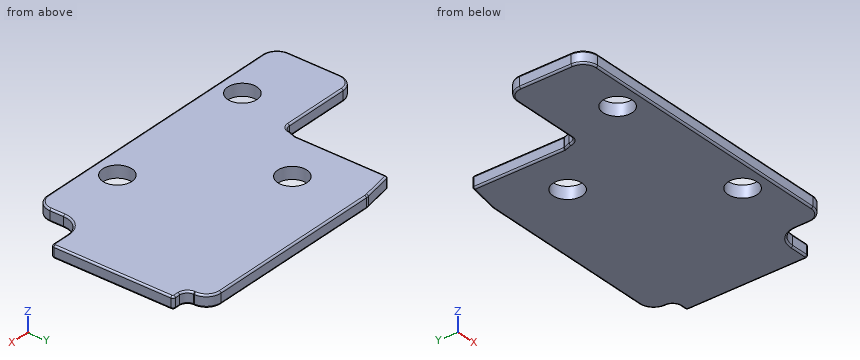
from build123d import *

# Parameters (mm, degrees)
SKETCH1_R           = 1.7
BOSS_EXTRUDE1_DEPTH = 1.4
FILLET1_R           = 0.2


with BuildPart() as part:
    # Sketch1 → Boss-Extrude1 (new body)
    with BuildSketch(Plane.XY):
        with BuildLine():
            Line((88.2, 306.15), (88.5, 306.997300304))
            Line((88.5, 306.997300304), (88.5, 317.666666667))
            Line((88.5, 317.666666667), (92.075260805, 318.322131148))
            ThreePointArc((92.075260805, 318.322131148), (92.227907414, 318.343018451), (92.381818182, 318.35))
            Line((92.381818182, 318.35), (113.2, 318.35))
            ThreePointArc((113.2, 318.35), (114.402081528, 317.852081528), (114.9, 316.65))
            Line((114.9, 316.65), (114.9, 316.55))
            ThreePointArc((114.9, 316.55), (115.163603897, 315.913603897), (115.8, 315.65))
            Line((115.8, 315.65), (116.4, 315.65))
            ThreePointArc((116.4, 315.65), (116.612132034, 315.562132034), (116.7, 315.35))
            Line((116.7, 315.35), (116.7, 301.75))
            ThreePointArc((116.7, 301.75), (116.612132034, 301.537867966), (116.4, 301.45))
            Line((116.4, 301.45), (114.4, 301.45))
            ThreePointArc((114.4, 301.45), (112.773654403, 300.776345597), (112.1, 299.15))
            Line((112.1, 299.15), (112.1, 297.55))
            ThreePointArc((112.1, 297.55), (111.602081528, 296.347918472), (110.4, 295.85))
            Line((110.4, 295.85), (79.6, 295.85))
            ThreePointArc((79.6, 295.85), (78.397918472, 296.347918472), (77.9, 297.55))
            Line((77.9, 297.55), (77.9, 303.55))
            ThreePointArc((77.9, 303.55), (78.397918472, 304.752081528), (79.6, 305.25))
            Line((79.6, 305.25), (87.3, 305.25))
            ThreePointArc((87.3, 305.25), (87.936396103, 305.513603897), (88.2, 306.15))
        make_face()
        with Locations((85.9, 298.65)):
            Circle(SKETCH1_R, mode=Mode.SUBTRACT)
        with Locations((103.8, 298.65)):
            Circle(SKETCH1_R, mode=Mode.SUBTRACT)
        with Locations((94, 311.05)):
            Circle(SKETCH1_R, mode=Mode.SUBTRACT)
    extrude(amount=BOSS_EXTRUDE1_DEPTH)

    # Fillet1
    fillet1_edges = [part.edges().sort_by_distance(p)[0] for p in [
        (88.35, 306.573650152, 1.4),
        (87.936396103, 305.513603897, 1.4),
        (83.45, 305.25, 1.4),
        (92.227907414, 318.343018451, 0),
        (102.790909091, 318.35, 0),
        (114.402081528, 317.852081528, 0),
        (114.9, 316.6, 0),
        (115.163603897, 315.913603897, 0),
        (116.1, 315.65, 0),
        (116.612132034, 315.562132034, 0),
        (116.7, 308.55, 0),
        (116.612132034, 301.537867966, 0),
        (115.4, 301.45, 0),
        (78.397918472, 304.752081528, 1.4),
        (112.773654403, 300.776345597, 0),
        (112.1, 298.35, 0),
        (111.602081528, 296.347918472, 0),
        (95, 295.85, 0),
        (78.397918472, 296.347918472, 0),
        (77.9, 300.55, 0),
        (78.397918472, 304.752081528, 0),
        (83.45, 305.25, 0),
        (87.936396103, 305.513603897, 0),
        (88.35, 306.573650152, 0),
        (77.9, 300.55, 1.4),
        (88.5, 312.331983485, 0),
        (90.287630402, 317.994398907, 0),
        (78.397918472, 296.347918472, 1.4),
        (95, 295.85, 1.4),
        (88.5, 306.997300304, 0.7),
        (88.5, 317.666666667, 0.7),
        (111.602081528, 296.347918472, 1.4),
        (112.1, 298.35, 1.4),
        (112.773654403, 300.776345597, 1.4),
        (90.287630402, 317.994398907, 1.4),
        (115.4, 301.45, 1.4),
        (116.612132034, 301.537867966, 1.4),
        (116.7, 308.55, 1.4),
        (116.612132034, 315.562132034, 1.4),
        (116.1, 315.65, 1.4),
        (115.163603897, 315.913603897, 1.4),
        (114.9, 316.6, 1.4),
        (114.402081528, 317.852081528, 1.4),
        (102.790909091, 318.35, 1.4),
        (92.227907414, 318.343018451, 1.4),
        (88.5, 312.331983485, 1.4),
    ]]
    fillet(fillet1_edges, radius=FILLET1_R)


solid = part.part
Could you check a few things on this model? Use its own coordinates, in mm. Give positions to 0.01 mm unless a question says otherwise; leave off trailing zeros. Order: outer loops, then holes, each group sorted by start corner. A loop starts at its lowest first (then second) coordinate and runs counter-clockwise, first axis right, second up. Notation, with made-up numbers: M 26.5,31.5 L 73.5,31.5 A14 ccw 73.5,58.5 Z; hole C 75.25,54 d3. An arc over 180 degrees is marked long. One line per question, with ' | ' between items.
1. I want a section at D-D (y = 311.05). List the corners of the cut face in (x, z) for me, and give its area (3 significant figures).
Results:
outline: M 88.5,0.2 A0.2 ccw 88.7,0 L 92.3,0 L 92.3,1.4 L 88.7,1.4 A0.2 ccw 88.5,1.2 Z; M 95.7,0 L 116.5,0 A0.2 ccw 116.7,0.2 L 116.7,1.2 A0.2 ccw 116.5,1.4 L 95.7,1.4 Z | area: 34.7 mm²
2. If I drill on line 1 (X direction, y = 298.65, z = 1); line 2 (Y direction, x = 103.8, z = 0.85); line 3 (Y direction, x = 85.9, z = 0.45), over which ranges is the centre line in solid material (lowest first)?
Results:
line 1: 77.9 to 84.2, 87.6 to 102.1, 105.5 to 112.1 | line 2: 295.85 to 296.95, 300.35 to 318.35 | line 3: 295.85 to 296.95, 300.35 to 305.25
3. I'm going to push a flat-ended pin straight in: pin 1 (2 mm diameter, centred on x = 103.8, y = 298.65, fed in from +Z). Where does the tip first touch, or does it pass through?
Results:
pin 1: through
4. I want a section at B-B (y = 298.65). List the corners of the cut face in (x, z) for me, and give its area (3 significant figures).
Results:
outline: M 77.9,0.2 A0.2 ccw 78.1,0 L 84.2,0 L 84.2,1.4 L 78.1,1.4 A0.2 ccw 77.9,1.2 Z; M 87.6,0 L 102.1,0 L 102.1,1.4 L 87.6,1.4 Z; M 105.5,0 L 111.9,0 A0.2 ccw 112.1,0.2 L 112.1,1.2 A0.2 ccw 111.9,1.4 L 105.5,1.4 Z | area: 38.3 mm²
5. I want a section at C-C (z = 0.45). List the corners of the cut face in (x, y) for me.
Results:
outline: M 77.9,297.55 A1.7 ccw 79.6,295.85 L 110.4,295.85 A1.7 ccw 112.1,297.55 L 112.1,299.15 A2.3 cw 114.4,301.45 L 116.4,301.45 A0.3 ccw 116.7,301.75 L 116.7,315.35 A0.3 ccw 116.4,315.65 L 115.8,315.65 A0.9 cw 114.9,316.55 L 114.9,316.65 A1.7 ccw 113.2,318.35 L 92.38,318.35 A1.7 ccw 92.08,318.32 L 88.66,317.7 A0.2 ccw 88.5,317.5 L 88.5,307.03 A0.2 cw 88.49,306.96 L 88.2,306.15 A0.9 cw 87.3,305.25 L 79.6,305.25 A1.7 ccw 77.9,303.55 Z; hole C 85.9,298.65 d3.4; hole C 94,311.05 d3.4; hole C 103.8,298.65 d3.4
6. I want a section at A-A (x = 85.9). List the corners of the cut face in (y, z) for me, and give its area (3 significant figures).
Results:
outline: M 295.85,0.2 A0.2 ccw 296.05,0 L 296.95,0 L 296.95,1.4 L 296.05,1.4 A0.2 ccw 295.85,1.2 Z; M 300.35,0 L 305.05,0 A0.2 ccw 305.25,0.2 L 305.25,1.2 A0.2 ccw 305.05,1.4 L 300.35,1.4 Z | area: 8.37 mm²
